Autodesk Inventor part; units mm, degrees
ref_plane "YZ Plane" through (0, 0, 0) normal (1, 0, 0) x (0, 1, 0)
ref_plane "XZ Plane" through (0, 0, 0) normal (0, 1, 0) x (-1, 0, 0)
ref_plane "XY Plane" through (0, 0, 0) normal (0, 0, 1) x (1, 0, 0)
sketch "Boceto1" plane through (0, 0, 0) normal (0, 1, 0) x (-1, 0, 0)
  line L0 (50.065, 16.445) -> (-50.065, 16.445)
  line L1 (-50.065, 16.445) -> (-50.065, -16.445)
  line L2 (-50.065, -16.445) -> (50.065, -16.445)
  line L3 (50.065, -16.445) -> (50.065, 16.445)
  point P0 (0, 0)
  dimension "q" = 100.13
  dimension "t" = 32.89
  dimension "d3" = 16.445
  dimension "d4" = 50.065
extrude "Extrusión1" add sketch "Boceto1" along normal blind 1.4
sketch "Boceto2" plane through (0, 1.4, 0) normal (0, 1, 0) x (1, 0, 0)
  circle A0 centre (-47.395, -13.855) radius 1
  circle A1 centre (-47.395, 13.855) radius 1
  line L0 (-50.065, -16.445) -> (50.065, -16.445)
  line L1 (50.065, 16.445) -> (-50.065, 16.445)
  line L2 (-50.065, 16.445) -> (-50.065, -16.445)
  circle A2 centre (47.705, -13.855) radius 1
  circle A3 centre (47.705, 13.855) radius 1
  line L3 (50.065, -16.445) -> (50.065, 16.445)
  point P0 (0, 0)
  dimension "d7" = 2
  dimension "d8" = 2
  dimension "v" = 2.59
  dimension "d10" = 2.59
  dimension "d11" = 2.67
  dimension "d12" = 2.67
  dimension "d13" = 2
  dimension "d14" = 2
  dimension "d15" = 2.59
  dimension "d16" = 2.59
  dimension "d17" = 2.36
  dimension "d18" = 2.36
extrude "Extrusión2" cut sketch "Boceto2" against normal blind 1.4 contours A0 | A1 | A2 | A3
sketch "Boceto3" plane through (0, 1.4, 0) normal (0, 1, 0) x (1, 0, 0)
  line L0 (-50.065, 16.445) -> (-50.065, -16.445)
  line L1 (-45.065, -5.0075) -> (-50.065, -5.0075)
  line L2 (-50.065, -5.0075) -> (-50.065, 4.9925)
  line L3 (-50.065, 4.9925) -> (-45.065, 4.9925)
  line L4 (-45.065, 4.9925) -> (-45.065, -5.0075)
  line L5 (8.065, -11.555) -> (21.065, -11.555)
  line L6 (21.065, -11.555) -> (21.065, 3.445)
  line L7 (21.065, 3.445) -> (8.065, 3.445)
  line L8 (8.065, 3.445) -> (8.065, -11.555)
  line L9 (50.065, -16.445) -> (50.065, 16.445)
  line L10 (50.065, 16.445) -> (-50.065, 16.445)
  line L11 (41.065, -6.555) -> (26.065, -6.555)
  line L12 (26.065, -6.555) -> (26.065, 5.445)
  line L13 (26.065, 5.445) -> (41.065, 5.445)
  line L14 (41.065, 5.445) -> (41.065, -6.555)
  point P0 (0, 0)
  dimension "d22" = 10
  dimension "d23" = 5
  dimension "d24" = 13
  dimension "d25" = 15
  dimension "d26" = 42
  dimension "d27" = 28
  dimension "d28" = 15
  dimension "d29" = 12
  dimension "d30" = 24
  dimension "d31" = 23
extrude "Extrusión3" add sketch "Boceto3" along normal blind 1.4
sketch "Boceto4" plane through (0, 2.8, 0) normal (0, 1, 0) x (1, 0, 0)
  point P0 (0, 0)
  point P1 (8.9547, -10.1632)
sketch "Boceto5" plane through (0, 2.8, 0) normal (0, 1, 0) x (1, 0, 0)
  line L0 (19.4822, 1.7557) -> (19.4822, -9.7421) construction
  line L1 (19.4822, -9.7421) -> (15.3355, -9.7421) construction
  line L2 (15.3355, -9.7421) -> (15.3355, 1.7557) construction
  line L3 (15.3355, 1.7557) -> (19.4822, 1.7557) construction
  point P0 (0, 0)
sketch "Boceto6" plane through (0, 2.8, 0) normal (0, 1, 0) x (1, 0, 0)
  line L0 (14.4245, 1.2531) -> (14.4245, -8.6603) construction
  line L1 (14.4245, -8.6603) -> (9.5235, -8.6603) construction
  line L2 (9.5235, -8.6603) -> (9.5235, 1.2531) construction
  line L3 (9.5235, 1.2531) -> (14.4245, 1.2531) construction
  point P0 (0, 0)
sketch "Boceto7" plane through (0, 1.4, 0) normal (0, 1, 0) x (1, 0, 0)
  circle A0 centre (44.565, -8.945) radius 2.5
  line L0 (50.065, -16.445) -> (50.065, 16.445)
  line L1 (-50.065, -16.445) -> (50.065, -16.445)
  point P0 (0, 0)
  dimension "d34" = 5
  dimension "d38" = 3
  dimension "d39" = 5
extrude "Extrusión4" cut sketch "Boceto7" against normal blind 1.4
sketch "Boceto8" plane through (0, 1.4, 0) normal (0, 1, 0) x (1, 0, 0)
  circle A0 centre (10.565, 14.8534) radius 1.5
  line L0 (50.065, -16.445) -> (50.065, 16.445)
  point P0 (0, 0)
  dimension "d42" = 3
  dimension "d43" = 41
extrude "Extrusión5" add sketch "Boceto8" along normal blind 1
equation "\"d10\" = v"
equation "\"d15\" = v"
equation "\"d16\" = v"
properties part number "tBeam"
For this review, take the finished solid that the model builds, in its own axes (mm). A direction names the side the tool comes from. Round coordinates to 2 decimals unless told otherwise and drop trailing zeros. Write each loop counter-clockwise with the first axis right and the second up, starting at its lowest first coordinate (ties: lowest second). Pieces come first, ordered by that corner, then holes. Notation, with made-up numbers: (32.5, 6.5) - (84.5, 6.5) arc R17 ccw to (84.5, 18.5) - close; hole circle Ø5 at (72, 27). An arc over 180 degrees is marked (long way). Use CSV: the item, a comma, the result in double quotes.
1) Clearance check with flat-ended pins moving along their axes: pin 1 Ø0.7 at (x, y) = (12, 2) entering from +Z (3 decimals); pin 2 Ø0.7 at (y, z) = (2, 7.5) entering from +X (3 decimals); pin 3 Ø2.5 at (x, z) = (47.705, 13.855) entering from +Y; pin 4 Ø1.6 at (x, z) = (47.705, -13.855) entering from -Y. State where each tip first meets the part, or that it passes through.
Conclusion:
pin 1,"stops at z = 11.555"
pin 2,"stops at x = 21.065"
pin 3,"stops at y = 1.4"
pin 4,"passes through"
2) For faces 1 (the flat face through (11, 2.4, -15)), 2 (the flat face through (14, 2.8, 4)), 3 (the cylindrical face through (11.996, 1.893, -14.403)), list the 3-axis set-ups (+Z, -Z, +X, -X, +Y, -Y) from which the entire face can be reached by the end or side of a thin tool; tool diameter is ignored.
Conclusion:
face 1,"-Z, +X, -X, +Y"
face 2,"+Z, -Z, +X, -X, +Y"
face 3,"+Y"
3) The part is to be moulded in two halves that separate along Z. For faces 4 (the cylindrical face through (48.24, 0.71, 13.01)), 5 (the flat face through (1, 0, 0)), say which applies: pulls with the +Z half, pulls with the -Z half, needs draft (parallel to the pull), parting line crosses it, or undercut.
Conclusion:
face 4,"undercut"
face 5,"needs draft"
4) Add section B-B on x = 38. Write out the cut boundary in (y, z) (3 decimals).
Conclusion:
outline,"(0, -16.445) - (1.4, -16.445) - (1.4, -5.445) - (2.8, -5.445) - (2.8, 6.555) - (1.4, 6.555) - (1.4, 16.445) - (0, 16.445) - close"
5) Wall thickness on line 1 along X through (y, z) = (2, -2) (3 decimals); line 2 along X through (y, z) = (0.6, -13) (3 decimals); line 3 along Z through (x, y) = (16.5, 2.4) (3 decimals): over which ranges is each line inside the solid? List them lowest first. Write a range as from..to.
Conclusion:
line 1,"x = -50.065..-45.065, 8.065..21.065, 26.065..41.065"
line 2,"x = -50.065..-47.914, -46.876..47.186, 48.224..50.065"
line 3,"z = -3.445..11.555"
6) Add section D-D on z = -9.5. Write out the cut boundary in (x, y) (3 decimals).
Conclusion:
outline,"(-50.065, 0) - (50.065, 0) - (50.065, 1.4) - (-50.065, 1.4) - close"
7) Add section C-C on x = 18. Write out the cut boundary in (y, z) (3 decimals), and give its area (3 significant figures).
Conclusion:
outline,"(0, -16.445) - (1.4, -16.445) - (1.4, -3.445) - (2.8, -3.445) - (2.8, 11.555) - (1.4, 11.555) - (1.4, 16.445) - (0, 16.445) - close"
area,"67.0 mm^2"
8) Add section A-A on z = 2.5. Write out the cut boundary in (x, y) (3 decimals), and give its area (3 significant figures).
Conclusion:
outline,"(-50.065, 0) - (50.065, 0) - (50.065, 1.4) - (41.065, 1.4) - (41.065, 2.8) - (26.065, 2.8) - (26.065, 1.4) - (21.065, 1.4) - (21.065, 2.8) - (8.065, 2.8) - (8.065, 1.4) - (-45.065, 1.4) - (-45.065, 2.8) - (-50.065, 2.8) - close"
area,"186 mm^2"
